from build123d import *

# Parameters (mm, degrees)
F0_R     = 30
F1_DEPTH = 40
F1_TAPER = 3
F2_T     = -0.85
F3_R     = 31.5488335059
F3_R_2   = 29.1488335059
F4_DEPTH = 1.2
F6_DEPTH = 32.5


with BuildPart() as f1:
    # F0 (on Top) → F1 (new body)
    with BuildSketch(Plane.XY):
        Circle(F0_R)
    extrude(amount=F1_DEPTH, taper=F1_TAPER)

    # F2
    f2_openings = [f1.faces().sort_by_distance(p)[0] for p in [
        (0, 0, 40),
        (0, 0, 0),
    ]]
    offset(amount=F2_T, openings=f2_openings)

    # F3 (on Top) → F4 (join)
    with BuildSketch(Plane.XY):
        Circle(F3_R)
        Circle(F3_R_2, mode=Mode.SUBTRACT)
    extrude(amount=F4_DEPTH)

    # F5 (on Front) → F6 (cut, symmetric)
    with BuildSketch(Plane.XZ):
        with BuildLine():
            Line((28.8675134595, 40), (-28.8675134595, 40))
            Line((-28.8675134595, 40), (-12.9903810568, 12.5))
            ThreePointArc((-12.9903810568, 12.5), (0, 5), (12.9903810568, 12.5))
            Line((12.9903810568, 12.5), (28.8675134595, 40))
        make_face()
    extrude(amount=F6_DEPTH, both=True, mode=Mode.SUBTRACT)


solid = f1.part
Model file for the job. Use its own axes, mm. A direction names the side the tool comes from. Give positions to 0.01 mm unless a question says otherwise; leave off trailing zeros. Order: outer loops, then holes, each group sorted by start corner. A loop starts at its lowest first (then second) coordinate and runs counter-clockwise, first axis right, second up. Notation, with made-up numbers: (79.25, 9) - (132.25, 9) arc R19 cw to (132.25, 40) - close; hole circle Ø2 at (54.5, 11.5). An arc over 180 degrees is marked (long way). Return JSON: item names as keys, results as strings.
1) Probe line 1 (X direction, y = -24, z = 2); line 2 (Y direction, x = 7.5, z = 2); line 3 (Z direction, x = 26, y = 17.5). List the from-to ranges inside material, lowest first. Write a range as from..to.
Geometry says:
{"line 1": "-17.82..-16.36, 16.36..17.82", "line 2": "-28.94..-28.06, 28.06..28.94", "line 3": "0..1.2"}
2) Cut at A-A, the plane z = 20.5. Give the cut face in (x, y), plus the area to 3 significant figures.
Geometry says:
{"outline": "(-17.61, -22.95) - (-17.61, -21.87) arc R28.07 cw to (-17.61, 21.87) - (-17.61, 22.95) arc R28.93 ccw to start; (17.61, -22.95) arc R28.93 ccw to (17.61, 22.95) - (17.61, 21.87) arc R28.07 cw to (17.61, -21.87) - close", "area": "87.8 mm²"}
3) Cut at C-C, the plane y = 0. Give the cut face in (x, z).
Geometry says:
{"outline": "(-31.55, 0) - (-29.15, 0) - (-27.2, 37.12) - (-27.98, 38.47) - (-29.94, 1.2) - (-31.55, 1.2) - close; (27.2, 37.12) - (29.15, 0) - (31.55, 0) - (31.55, 1.2) - (29.94, 1.2) - (27.98, 38.47) - close"}
4) Pull direction X, two halves, no side cores. Call faces 4 (the conical face through (-29.136, 1.282, 15.955)), 5 (the flat face through (9, -28, 0)), 6 (the cylindrical face through (-0.1, -29.2, 5)): pulls with the +X half, pulls with the -X half, needs draft (parallel to the pull), parting line crosses it, or undercut.
Geometry says:
{"face 4": "parting line crosses it", "face 5": "needs draft", "face 6": "undercut"}
5) Cut at B-B, the plane x = 0. Give the cut face in (y, z).
Geometry says:
{"outline": "(-31.55, 0) - (-29.15, 0) - (-28.89, 5) - (-29.74, 5) - (-29.94, 1.2) - (-31.55, 1.2) - close; (28.89, 5) - (29.15, 0) - (31.55, 0) - (31.55, 1.2) - (29.94, 1.2) - (29.74, 5) - close"}
6) Cut at D-D, the plane z = 15. Give the cut face in (x, y), plus the area to 3 significant figures.
Geometry says:
{"outline": "(-14.43, -25.4) - (-14.43, -24.42) arc R28.36 cw to (-14.43, 24.42) - (-14.43, 25.4) arc R29.21 ccw to start; (14.43, -25.4) arc R29.21 ccw to (14.43, 25.4) - (14.43, 24.42) arc R28.36 cw to (14.43, -24.42) - close", "area": "102 mm²"}
7) Flat gauge pins, fed straight in: P1, Ø6, axis at x = 15.5, y = 23, coming from the +Z side; P2, Ø1.5, axis at y = 3, z = 26, coming from the +X side; P3, Ø4, axis at y = 19.5, z = 24.5, coming from the +X side; P4, Ø12, axis at x = -10.5, z = 26.5, coming from the +Y side. Where does each tip first touch, or does it go through?
Geometry says:
{"P1": "z = 21.87", "P2": "x = 28.56", "P3": "x = 22.77", "P4": "through"}
8) 3-axis set-ups, long thin cutter, end or side, ignore diameter. For faces 1 (the flat face through (27.12, 3.78, 36.97)), 2 (the flat face through (-24, -19, 1.2)), 3 (the conical face through (-28.35, 1.25, 14.69)): which of +Z, -Z, +X, -X, +Y, -Y reach the whole face in a straight line?
Geometry says:
{"face 1": "+Z, +Y, -Y", "face 2": "+Z", "face 3": "-Z"}
